Geometry: final body of the model. Coordinates: model frame, mm. Face numbers are marked on the shaded views. Coordinates: 2 decimals unless noted, no trailing zeros. Order: outer loops, then holes, each group sorted by start corner. A loop starts at its lowest first (then second) coordinate and runs counter-clockwise, first axis right, second up. Notation, with made-up numbers: (52, -13) - (59, -13) arc R7 ccw to (59, -5) - close; hole circle Ø6 at (88.5, 64). An arc over 180 degrees is marked (long way). Use a Markdown table: item, result. Add a question column.
```python
from build123d import *

# Parameters (mm, degrees)
BOSS_EXTRUDE1_DEPTH = 7.85
SKETCH18_W          = 3.3
SKETCH18_H          = 2.5
CUT_EXTRUDE10_DEPTH = 43.3
SKETCH19_W          = 3.3
SKETCH19_H          = 2.5
CUT_EXTRUDE11_DEPTH = 43.3
SKETCH20_W          = 6.221233688
SKETCH20_H          = 2.5
CUT_EXTRUDE12_DEPTH = 57.710616844
SKETCH21_W          = 6.221233688
SKETCH21_H          = 2.5
CUT_EXTRUDE13_DEPTH = 57.710616844
SKETCH22_R          = 2.5
CUT_EXTRUDE14_DEPTH = 6.35
CUT_EXTRUDE15_DEPTH = 14.2
FILLET8_R           = 6


with BuildPart() as part:
    # Sketch1 → Boss-Extrude1 (new body)
    with BuildSketch(Plane(origin=(0, 0, 0), x_dir=(1, 0, 0), z_dir=(0, 1, 0))):
        Polygon((-21.15, 16.750923472), (-16.750923472, 21.15), (16.750923472, 21.15), (21.15, 16.750923472), (21.15, -16.750923472), (16.750923472, -21.15), (-16.750923472, -21.15), (-21.15, -16.750923472), align=None)
    boss_extrude1 = extrude(amount=BOSS_EXTRUDE1_DEPTH)

    # Sketch18 → Cut-Extrude10 (cut, through all)
    with BuildSketch(Plane.XY.offset(21.15)):
        with Locations((15.100923472, 6.6)):
            Rectangle(SKETCH18_W, SKETCH18_H)
        with Locations((-15.100923472, 6.6)):
            Rectangle(SKETCH18_W, SKETCH18_H)
    cut_extrude10 = extrude(amount=-CUT_EXTRUDE10_DEPTH, mode=Mode.SUBTRACT)

    # Sketch19 → Cut-Extrude11 (cut, through all)
    with BuildSketch(Plane(origin=(21.15, 0, 0), x_dir=(0, 0, -1), z_dir=(1, 0, 0))):
        with Locations((-15.100923472, 6.6)):
            Rectangle(SKETCH19_W, SKETCH19_H)
        with Locations((15.100923472, 6.6)):
            Rectangle(SKETCH19_W, SKETCH19_H)
    cut_extrude11 = extrude(amount=-CUT_EXTRUDE11_DEPTH, mode=Mode.SUBTRACT)

    # Sketch20 → Cut-Extrude12 (cut, through all)
    with BuildSketch(Plane(origin=(18.950461736, 0, 18.950461736), x_dir=(0.707106781, 0, -0.707106781), z_dir=(0.707106781, 0, 0.707106781))):
        with Locations((0, 6.6)):
            Rectangle(SKETCH20_W, SKETCH20_H)
    cut_extrude12 = extrude(amount=-CUT_EXTRUDE12_DEPTH, mode=Mode.SUBTRACT)

    # Sketch21 → Cut-Extrude13 (cut, through all)
    with BuildSketch(Plane(origin=(-18.950461736, 0, 18.950461736), x_dir=(0.707106781, 0, 0.707106781), z_dir=(-0.707106781, 0, 0.707106781))):
        with Locations((0, 6.6)):
            Rectangle(SKETCH21_W, SKETCH21_H)
    cut_extrude13 = extrude(amount=-CUT_EXTRUDE13_DEPTH, mode=Mode.SUBTRACT)

    # Sketch22 → Cut-Extrude14 (cut, through all)
    with BuildSketch(Plane(origin=(0, 5.35, 0), x_dir=(1, 0, 0), z_dir=(0, 1, 0))):
        Circle(SKETCH22_R)
    cut_extrude14 = extrude(amount=-CUT_EXTRUDE14_DEPTH, mode=Mode.SUBTRACT)

    # Mirror1: Boss-Extrude1, Cut-Extrude10, Cut-Extrude11, Cut-Extrude12, Cut-Extrude13, Cut-Extrude14 across plane
    add(boss_extrude1.mirror(Plane(origin=(0, 0, 0), x_dir=(0, 0, 1), z_dir=(0, -1, 0))))
    add(cut_extrude10.mirror(Plane(origin=(0, 0, 0), x_dir=(0, 0, 1), z_dir=(0, -1, 0))), mode=Mode.SUBTRACT)
    add(cut_extrude11.mirror(Plane(origin=(0, 0, 0), x_dir=(0, 0, 1), z_dir=(0, -1, 0))), mode=Mode.SUBTRACT)
    add(cut_extrude12.mirror(Plane(origin=(0, 0, 0), x_dir=(0, 0, 1), z_dir=(0, -1, 0))), mode=Mode.SUBTRACT)
    add(cut_extrude13.mirror(Plane(origin=(0, 0, 0), x_dir=(0, 0, 1), z_dir=(0, -1, 0))), mode=Mode.SUBTRACT)
    add(cut_extrude14.mirror(Plane(origin=(0, 0, 0), x_dir=(0, 0, 1), z_dir=(0, -1, 0))), mode=Mode.SUBTRACT)

    # Sketch23 → Cut-Extrude15 (cut, through all)
    with BuildSketch(Plane(origin=(0, 5.35, 0), x_dir=(1, 0, 0), z_dir=(0, 1, 0))):
        Polygon((-21.15, -14.432485579), (-14.432485579, -21.15), (-16.750923472, -21.15), (-21.15, -16.750923472), align=None)
        Polygon((-21.15, 14.432485579), (-14.432485579, 21.15), (-16.750923472, 21.15), (-21.15, 16.750923472), align=None)
        Polygon((14.432485579, 21.15), (21.15, 14.432485579), (21.15, 16.750923472), (16.750923472, 21.15), align=None)
        Polygon((14.432485579, -21.15), (21.15, -14.432485579), (21.15, -16.750923472), (16.750923472, -21.15), align=None)
    extrude(amount=-CUT_EXTRUDE15_DEPTH, mode=Mode.SUBTRACT)

    # Fillet8
    fillet8_edges = [part.edges().sort_by_distance(p)[0] for p in [
        (14.432485579, 0, -21.15),
        (21.15, 0, -14.432485579),
        (-21.15, 0, -14.432485579),
        (-14.432485579, 0, -21.15),
        (-14.432485579, 0, 21.15),
        (-21.15, 0, 14.432485579),
        (21.15, 0, 14.432485579),
        (14.432485579, 0, 21.15),
    ]]
    fillet(fillet8_edges, radius=FILLET8_R)


solid = part.part
```
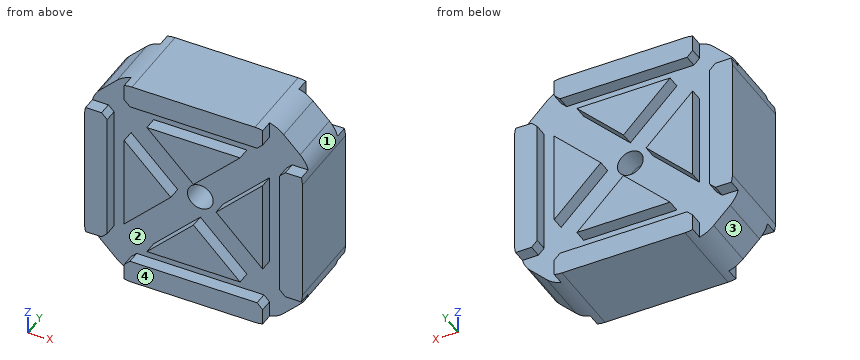
1) Pin query (flat end, axial travel): pin 1 (3 mm diameter, centred on x = 19.5, y = -7, fed in from +Z); pin 2 (0.8 mm diameter, centred on y = -7, z = -19.5, fed in from -X); pin 3 (2 mm diameter, centred on x = -19, y = 7, fed in from -Z). Return the tip coordinate at first contact, or that it passes through.
2) Section A-A (y = -1.5). Return loops of the section in (x, z), then the cut area to 3 significant figures.
3) Section D-D (z = 15). Return loops of the section in (x, y).
4) Draft query along X for the marked faces 1, 2, 3 and 4. Return one class per face: pulls with the +X half, pulls with the -X half, needs draft (parallel to the pull), parting line crosses it, or undercut.
5) Ray query, line 1 along Z through (x, y) = (0, -1.6); line 2 along Y through (x, z) = (0, -13.5). Return the intervals inside material, ascending.
Values follow:
| question | item | result |
|---|---|---|
| 1 | pin 1 | stops at z = 13.45 |
| 1 | pin 2 | stops at x = -13.45 |
| 1 | pin 3 | stops at z = -13.45 |
| 2 | outline | (-21.15, -11.95) arc R6 ccw to (-19.39, -16.19) - (-16.19, -19.39) arc R6 ccw to (-11.95, -21.15) - (11.95, -21.15) arc R6 ccw to (16.19, -19.39) - (19.39, -16.19) arc R6 ccw to (21.15, -11.95) - (21.15, 11.95) arc R6 ccw to (19.39, 16.19) - (16.19, 19.39) arc R6 ccw to (11.95, 21.15) - (-11.95, 21.15) arc R6 ccw to (-16.19, 19.39) - (-19.39, 16.19) arc R6 ccw to (-21.15, 11.95) - close; hole circle Ø5 at (0, 0) |
| 2 | area | 1,670 mm² |
| 3 | outline | (-20.32, -5.35) - (20.32, -5.35) - (20.32, 5.35) - (-20.32, 5.35) - close |
| 4 | face 1 | pulls with the +X half |
| 4 | face 2 | undercut |
| 4 | face 3 | pulls with the -X half |
| 4 | face 4 | needs draft |
| 5 | line 1 | z = -21.15 to -2.5, 2.5 to 21.15 |
| 5 | line 2 | y = -5.35 to 5.35 |
